from build123d import *

# Parameters (mm, degrees)
SKETCH1_W           = 20
SKETCH1_H           = 46.001723395
BOSS_EXTRUDE1_DEPTH = 100
SKETCH8_W           = 15.5
SKETCH8_H           = 15
BOSS_EXTRUDE2_DEPTH = 57
SKETCH10_R          = 5.95
CUT_EXTRUDE1_DEPTH  = 51
SKETCH11_W          = 10
SKETCH11_H          = 18.6
BOSS_EXTRUDE3_DEPTH = 60
FILLET2_R           = 1


with BuildPart() as part:
    # Sketch1 → Boss-Extrude1 (new body)
    with BuildSketch(Plane(origin=(0, 0, 0), x_dir=(1, 0, 0), z_dir=(0, 1, 0))):
        Polygon((-17.351649908, 20.312727502), (-57.351649908, -25.688995893), (-17.351649908, -25.688995893), align=None)
        with Locations((-7.351649908, -2.688134195)):
            Rectangle(SKETCH1_W, SKETCH1_H)
    extrude(amount=-BOSS_EXTRUDE1_DEPTH)

    # Sketch8 → Boss-Extrude2 (add)
    with BuildSketch(Plane(origin=(2.648350092, 0, 0), x_dir=(0, 0, -1), z_dir=(1, 0, 0))):
        with Locations((-33.438995893, -15.35)):
            Rectangle(SKETCH8_W, SKETCH8_H)
        with Locations((-33.438995893, -38.45)):
            Rectangle(SKETCH8_W, SKETCH8_H)
        with Locations((-33.438995893, -61.55)):
            Rectangle(SKETCH8_W, SKETCH8_H)
        with Locations((-33.438995893, -84.65)):
            Rectangle(SKETCH8_W, SKETCH8_H)
    extrude(amount=-BOSS_EXTRUDE2_DEPTH)

    # Sketch10 → Cut-Extrude1 (cut)
    with BuildSketch(Plane(origin=(2.648350092, 0, 0), x_dir=(0, 0, -1), z_dir=(1, 0, 0))):
        with Locations((-33.438995893, -15.35)):
            Circle(SKETCH10_R)
        with Locations((-33.438995893, -38.45)):
            Circle(SKETCH10_R)
        with Locations((-33.438995893, -61.55)):
            Circle(SKETCH10_R)
        with Locations((-33.438995893, -84.65)):
            Circle(SKETCH10_R)
    extrude(amount=-CUT_EXTRUDE1_DEPTH, mode=Mode.SUBTRACT)

    # Sketch11 → Boss-Extrude3 (add)
    with BuildSketch(Plane(origin=(2.648350092, 0, 0), x_dir=(0, 0, -1), z_dir=(1, 0, 0))):
        with Locations((-46.188995893, -15.35)):
            Rectangle(SKETCH11_W, SKETCH11_H)
        with Locations((-46.188995893, -38.45)):
            Rectangle(SKETCH11_W, SKETCH11_H)
        with Locations((-46.188995893, -84.65)):
            Rectangle(SKETCH11_W, SKETCH11_H)
        with Locations((-46.188995893, -61.55)):
            Rectangle(SKETCH11_W, SKETCH11_H)
    extrude(amount=-BOSS_EXTRUDE3_DEPTH)

    # Fillet2
    fillet2_edges = [part.edges().sort_by_distance(p)[0] for p in [
        (-57.351649908, -50, 25.688995893),
    ]]
    fillet(fillet2_edges, radius=FILLET2_R)


solid = part.part
Model file for the job. Use its own axes, mm. A direction names the side the tool comes from. Give positions to 0.01 mm unless a question says otherwise; leave off trailing zeros. Loops run counter-clockwise (first coordinate to the right, second up) from the corner with the lowest first, then second, coordinate; pieces in that order, holes last. Notation, with made-up numbers: (68.5, -14.75) -> (112.5, -14.75) arc R21 cw to (112.5, -4.75) -> close; hole circle Ø7 at (15, 72). An arc over 180 degrees is marked (long way). Use a Markdown table: item, result. Add a question column.
(1) Drop flat-ended pins along their axis: pin 1 Ø8 at (x, z) = (-15.5, 45.5) entering from +Y; pin 2 Ø1.5 at (x, y) = (-40.5, -26) entering from +Z; pin 3 Ø1.5 at (x, y) = (-21, -45.5) entering from -Z. Give the stop position or say it passes through.
(2) Mould opens along Y. For faces 1 (the flat face through (-27, -29.15, 46)), 2 (the flat face through (-21, -100, 7)), 3 (the flat face through (-54.352, -15, 34)), 4 (the flat face through (-27, -6.05, 46)) say: +Y half, -Y half, draft (parallel to the pull), parting line (faces both ways), or undercut.
(3) Slice it at B-B on y = -38.45. List the corners of the cut face in (x, z).
(4) Wall check: line 1 along Y through (x, z) = (-52.5, 35); line 2 along Y through (x, z) = (-25, 47); line 3 along Z through (x, y) = (-7, -15). Give the ranges that are in metal, low to high.
(5) Slice it at A-A on z = 35. Give the number of separate pieces and of enclosed holes in the cut face, and give its area (3 significant figures).
(6) Slice it at D-D on z = 22.5. List the corners of the cut face in (x, y), and give its area (3 significant figures).
(7) Tool access for faces 5 (the flat face through (-25, -22.85, 34)), 6 (the flat face through (-27, -52.25, 46)), 7 (the flat face through (-54.352, -38, 34)), 8 (the flat face through (-27, -93.95, 46)): list every direction of +Z, -Z, +X, -X, +Y, -Y with a clear straight run to the whole face (end or side of a thin tool).
Filled sheet:
| question | item | result |
|---|---|---|
| 1 | pin 1 | y = -6.05 |
| 1 | pin 2 | z = 25.69 |
| 1 | pin 3 | z = -16.98 |
| 2 | face 1 | undercut |
| 2 | face 2 | -Y half |
| 2 | face 3 | draft |
| 2 | face 4 | +Y half |
| 3 | outline | (-57.35, 41.19) -> (-54.35, 41.19) -> (-54.35, 25.69) -> (-55.16, 25.69) arc R1 ccw to (-55.91, 24.03) -> (-17.35, -20.31) -> (2.65, -20.31) -> (2.65, 27.49) -> (-48.35, 27.49) -> (-48.35, 39.39) -> (2.65, 39.39) -> (2.65, 51.19) -> (-57.35, 51.19) -> close |
| 4 | line 1 | -92.15 to -77.15, -69.05 to -54.05, -45.95 to -30.95, -22.85 to -7.85 |
| 4 | line 2 | -93.95 to -75.35, -70.85 to -52.25, -47.75 to -29.15, -24.65 to -6.05 |
| 4 | line 3 | -20.31 to 27.5, 39.38 to 51.19 |
| 5 | separate pieces | 4 |
| 5 | enclosed holes | 0 |
| 5 | area | 1,080 mm2 |
| 6 | outline | (-54.58, -100) -> (2.65, -100) -> (2.65, 0) -> (-54.58, 0) -> close |
| 6 | area | 5,720 mm2 |
| 7 | face 5 | +X, -X |
| 7 | face 6 | +Z, +X, -X |
| 7 | face 7 | -X, +Y, -Y |
| 7 | face 8 | +Z, +X, -X, -Y |
